Input: part model. Units: mm. Frame: model coordinates. A direction names the side the tool comes from. Coordinates: 2 decimals unless noted, no trailing zeros. Answer as a JSON object with one key per item and string values. Group by question number.
from build123d import *

# Parameters (mm, degrees)
BOSS_EXTRUDE1_DEPTH = 431.8
SKETCH4_W           = 15.875
SKETCH4_H           = 25.4
CUT_EXTRUDE1_DEPTH  = 6.35
SKETCH5_W           = 1.5875
SKETCH5_H           = 25.4
CUT_EXTRUDE2_DEPTH  = 6.35
SKETCH6_R           = 1.4224
CUT_EXTRUDE3_DEPTH  = 5.08
CUT_EXTRUDE4_START  = -2.54
CUT_EXTRUDE4_DEPTH  = 2.54
SKETCH8_R           = 1.4224
CUT_EXTRUDE5_DEPTH  = 5.08
SKETCH9_W           = 28.861002292
SKETCH9_H           = 547.524656259
CUT_EXTRUDE6_DEPTH  = 30.48
CUT_EXTRUDE7_START  = -3.175
CUT_EXTRUDE7_DEPTH  = 3.175


# Read off the part's stored shape, not the designer's step: Cut-Extrude7
with BuildPart() as part:
    # Sketch2 → Boss-Extrude1 (new body)
    with BuildSketch(Plane(origin=(0, 0, 0), x_dir=(1, 0, 0), z_dir=(0, 1, 0))):
        with BuildLine():
            Line((0, 0), (19.05, 0))
            Line((19.05, 0), (19.05, 1.5875))
            ThreePointArc((19.05, 1.5875), (18.585032015, 2.710032015), (17.4625, 3.175))
            Line((17.4625, 3.175), (4.7625, 3.175))
            ThreePointArc((4.7625, 3.175), (3.639967985, 3.639967985), (3.175, 4.7625))
            Line((3.175, 4.7625), (3.175, 17.4625))
            ThreePointArc((3.175, 17.4625), (2.710032015, 18.585032015), (1.5875, 19.05))
            Line((1.5875, 19.05), (0, 19.05))
            Line((0, 19.05), (0, 0))
        make_face()
    extrude(amount=BOSS_EXTRUDE1_DEPTH)

    # Sketch4 → Cut-Extrude1 (cut)
    with BuildSketch(Plane(origin=(3.175, 0, 0), x_dir=(0, 0, -1), z_dir=(1, 0, 0))):
        with Locations((11.1125, 419.1)):
            Rectangle(SKETCH4_W, SKETCH4_H)
    extrude(amount=-CUT_EXTRUDE1_DEPTH, mode=Mode.SUBTRACT)

    # Sketch5 → Cut-Extrude2 (cut)
    with BuildSketch(Plane.ZY.offset(-3.175)):
        with Locations((-3.96875, 419.1)):
            Rectangle(SKETCH5_W, SKETCH5_H)
    extrude(amount=-CUT_EXTRUDE2_DEPTH, mode=Mode.SUBTRACT)

    # Sketch6 → Cut-Extrude3 (cut)
    with BuildSketch(Plane(origin=(3.175, 0, 0), x_dir=(0, 0, -1), z_dir=(1, 0, 0))):
        with Locations((11.1125, 109.5375)):
            Circle(SKETCH6_R)
        with Locations((11.1125, 203.2)):
            Circle(SKETCH6_R)
        with Locations((11.1125, 296.8625)):
            Circle(SKETCH6_R)
        with Locations((11.1125, 11.1125)):
            Circle(SKETCH6_R)
        with Locations((11.1125, 395.2875)):
            Circle(SKETCH6_R)
    extrude(amount=-CUT_EXTRUDE3_DEPTH, mode=Mode.SUBTRACT)

    # Sketch7 → Cut-Extrude4 (cut)
    with BuildSketch(Plane(origin=(0, 431.8, 0), x_dir=(1, 0, 0), z_dir=(0, 1, 0)).offset(CUT_EXTRUDE4_START)):
        with BuildLine():
            Line((17.4625, 3.175), (0, 3.175))
            Line((0, 3.175), (0, 0))
            Line((0, 0), (19.05, 0))
            Line((19.05, 0), (19.05, 1.5875))
            ThreePointArc((19.05, 1.5875), (18.585032015, 2.710032015), (17.4625, 3.175))
        make_face()
    extrude(amount=CUT_EXTRUDE4_DEPTH, mode=Mode.SUBTRACT)

    # Sketch8 → Cut-Extrude5 (cut)
    with BuildSketch(Plane(origin=(0, 0, -3.175), x_dir=(-1, 0, 0), z_dir=(0, 0, -1))):
        with Locations((-9.525, 419.735)):
            Circle(SKETCH8_R)
    extrude(amount=-CUT_EXTRUDE5_DEPTH, mode=Mode.SUBTRACT)


with BuildPart() as body_2:
    # Mirror3: mirrored copy
    add(part.part.mirror(Plane.XY.offset(2.54)))

    # Cut-Extrude7 outline → Cut-Extrude7 (cut)
    with BuildSketch(Plane.XY.offset(8.255).offset(CUT_EXTRUDE7_START)):
        with BuildLine():
            ThreePointArc((0, 419.735), (2.789807909, 426.470192091), (9.525, 429.26))
            Line((9.525, 429.26), (0, 429.26))
            Line((0, 429.26), (0, 419.735))
        make_face()
        with BuildLine():
            ThreePointArc((9.525, 429.26), (16.260192091, 426.470192091), (19.05, 419.735))
            Line((19.05, 419.735), (19.05, 429.26))
            Line((19.05, 429.26), (9.525, 429.26))
        make_face()
    extrude(amount=CUT_EXTRUDE7_DEPTH, mode=Mode.SUBTRACT)


with BuildPart() as part_1:
    add(part.part)

    # Sketch9 → Cut-Extrude6 (cut)
    with BuildSketch(Plane.XY.offset(2.54)):
        with Locations((7.805746781, 195.778589833)):
            Rectangle(SKETCH9_W, SKETCH9_H)
    extrude(amount=-CUT_EXTRUDE6_DEPTH, mode=Mode.SUBTRACT)


solid = body_2.part
Q1. Line query: line 1 (X direction, y = 129, z = 19.25) (3 decimals); line 2 (Z direction, x = 9, y = 45) (3 decimals); line 3 (Y direction, x = 3, z = 15). Output: solid intervals per line, ascending. Write a range as from..to.
Q2. Access query for faces 1 (the flat face through (0, 207, 15)), 2 (the flat face through (3.175, 200, 16)). Directions: +Z, -Z, +X, -X, +Y, -Y. A direction counts if a zero-diameter tool reaches every point of the face in a straight line with its end or side. Return the directions, or none.
Q3. Pin query (flat end, axial travel): pin 1 Ø5 at (y, z) = (343, 9.5) entering from +X; pin 2 Ø1.7 at (y, z) = (109.54, 16.19) entering from -X; pin 3 Ø10 at (x, z) = (7.5, 18.5) entering from +Y; pin 4 Ø6.5 at (y, z) = (173.5, 17) entering from +X (3 decimals). Return the tip coordinate at first contact, or that it passes through.
Filled in:
{
 "1": {"line 1": "0..3.175", "line 2": "5.08..8.255", "line 3": "0..10.34, 11.89..108.76, 110.31..202.42, 203.98..296.09, 297.64..394.51, 396.06..406.4"},
 "2": {"face 1": "+Z, -Z, -X, +Y, -Y", "face 2": "+Z, +X, +Y, -Y"},
 "3": {"pin 1": "x = 19.01", "pin 2": "through", "pin 3": "y = 406.4", "pin 4": "x = 3.175"}
}
